```python
from build123d import *

# Parameters (mm, degrees)
SKETCH_1_R      = 3.375
SKETCH_1_R_2    = 2.5
EXTRUDE_1_DEPTH = 100


with BuildPart() as part:
    # 草图1 → 凸台-拉伸1 (new body)
    with BuildSketch(Plane.XY):
        Polygon((0, 0), (14.9, 0), (14.9, 1), (15.75, 1), (15.75, 4.5), (10, 4.5), (10, 8.040202025), (15.959797975, 14), (24.040202025, 14), (30, 8.040202025), (30, 4.5), (24.25, 4.5), (24.25, 1), (25.1, 1), (25.1, 0), (40, 0), (40, 14.9), (39, 14.9), (39, 15.4), (35.5, 15.4), (35.5, 12.4), (37, 12.4), (37, 9.7), (32.3, 9.7), (26, 16), (26, 24), (29.5, 27.5), (35.5, 27.5), (35.5, 24.6), (39, 24.6), (39, 25.1), (40, 25.1), (40, 30), (25.1, 30), (25.1, 29), (24.25, 29), (24.25, 26), (15.75, 26), (15.75, 29), (14.9, 29), (14.9, 30), (0, 30), (0, 25.1), (1, 25.1), (1, 24.6), (4.5, 24.6), (4.5, 27.5), (10.5, 27.5), (14, 24), (14, 16), (7.7, 9.7), (3, 9.7), (3, 12.4), (4.5, 12.4), (4.5, 15.4), (1, 15.4), (1, 14.9), (0, 14.9), align=None)
        with Locations((20, 20)):
            Circle(SKETCH_1_R, mode=Mode.SUBTRACT)
        with Locations((35, 5)):
            Circle(SKETCH_1_R_2, mode=Mode.SUBTRACT)
        with Locations((5, 5)):
            Circle(SKETCH_1_R_2, mode=Mode.SUBTRACT)
    extrude(amount=EXTRUDE_1_DEPTH)


solid = part.part
```
Read the model definition and answer for the solid it produces. Units are mm, in the model's axes. A direction names the side the tool comes from. Give positions to 0.01 mm unless a question says otherwise; leave off trailing zeros. Loops run counter-clockwise (first coordinate to the right, second up) from the corner with the lowest first, then second, coordinate; pieces in that order, holes last.
Item 1: This flat-tipped pin is pushed along its axis until it touches: pin 1 Ø2.5 at (x, z) = (18.5, 32) entering from -Y. Where does it stop, or does it pass through?
Item 2: The mould has two halves that part along X. Classify faces 4 (the flat face through (40, 28, 49)), 5 (the flat face through (29, 13, 49)), 6 (the flat face through (32, 0, 49)), 7 (the flat face through (20, 14, 49)): released by +X, released by -X, zero draft, split by the parting line, or undercut.
Item 3: Find the intervals of material crossed by line 1 along Y through (x, z) = (35, 55); line 2 along Y through (x, z) = (20, 65) (3 decimals); line 3 along Y through (x, z) = (28, 73), in increasing order.
Item 4: The part is cut by section B-B (y = 20). Write down the section's boundary in (x, z) (3 decimals), and give its area (3 significant figures).
Item 5: The part is cut by section C-C (z = 62). Give the number of separate pieces and of enclosed holes in the cut face, and give its area (3 significant figures).
Item 6: For faces 1 (the flat face through (37, 24.6, 49)), 2 (the flat face through (20, 26, 49)), 3 (the flat face through (5, 9.7, 49)), determine the directions among +Z, -Z, +X, -X, +Y, -Y from which every point of the face is accessible in a straight line to the end or side of a thin tool.
Item 7: The part is cut by section A-A (x = 31). Write down the section's boundary in (y, z).
Taken from the geometry:
1. pin 1: stops at y = 14
2. face 4: released by +X
2. face 5: undercut
2. face 6: zero draft
2. face 7: undercut
3. line 1: y = 0 to 2.5, 7.5 to 9.7, 27.5 to 30
3. line 2: y = 14 to 16.625, 23.375 to 26
3. line 3: y = 0 to 4.5, 10.04 to 14, 26 to 30
4. outline: (14, 0) - (16.625, 0) - (16.625, 100) - (14, 100) - close; (23.375, 0) - (26, 0) - (26, 100) - (23.375, 100) - close
4. area: 525 mm2
5. separate pieces: 1
5. enclosed holes: 3
5. area: 516 mm2
6. face 1: +Z, -Z, +X
6. face 2: +Z, -Z, +Y
6. face 3: +Z, -Z
7. outline: (0, 0) - (11, 0) - (11, 100) - (0, 100) - close; (27.5, 0) - (30, 0) - (30, 100) - (27.5, 100) - close
